Read the model definition and answer for the solid it produces. Units are mm, in the model's axes. Face numbers are marked on the shaded views. A direction names the side the tool comes from. Coordinates: 2 decimals unless noted, no trailing zeros. Write each loop counter-clockwise with the first axis right and the second up, starting at its lowest first coordinate (ties: lowest second). Pieces come first, ordered by that corner, then holes.
1) Determine the mould class of the marked faces 3, 4, 5 and 6 for opening direction X: +X half, -X half, draft (parallel to the pull), parting line (faces both ways), or undercut.
2) Find the intervals of material crossed by line 1 (X direction, y = 1.85, z = -8); line 2 (Z direction, x = 8, y = 1.75); line 3 (Z direction, x = 8, y = -2.25), in increasing order.
3) The part is cut by section D-D (z = -2.75). Determine the outline of the cut face in (x, y), then the cut area to 3 significant figures.
4) Which of the six approach directions +Z, -Z, +X, -X, +Y, -Y give full straight-line access (tool end or side, diameter ignored) to the marked faces 1 and 2?
5) The part is cut by section A-A (z = -8). Determine the outline of the cut face in (x, y), then the cut area to 3 significant figures.
6) The part is cut by section B-B (x = 8). Determine the outline of the cut face in (y, z), then the cut area to 3 significant figures.
7) This flat-tipped pin is pushed along its axis until it touches: pin 1 Ø2 at (x, z) = (5.5, -8.5) entering from +Y. Where does it stop, or does it pass through?
8) The part is cut by section C-C (y = -3.75). Determine the outline of the cut face in (x, z).
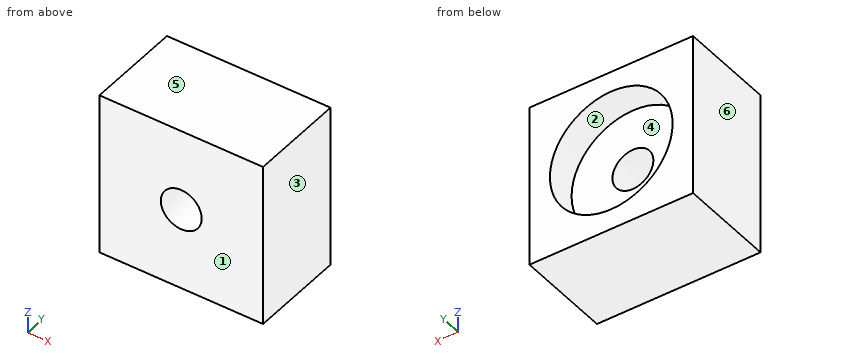
from build123d import *

# Parameters (mm, degrees)
SKETCH1_W           = 16
SKETCH1_H           = 16
SKETCH1_R           = 6
BOSS_EXTRUDE1_DEPTH = 3
SKETCH2_W           = 16
SKETCH2_H           = 16
BOSS_EXTRUDE2_DEPTH = 6.35
SKETCH3_R           = 2
CUT_EXTRUDE1_DEPTH  = 6.35


with BuildPart() as part:
    # Sketch1 → Boss-Extrude1 (new body)
    with BuildSketch(Plane(origin=(0, 0, 0), x_dir=(1, 0, 0), z_dir=(0, 1, 0))):
        with Locations((8, 8)):
            Rectangle(SKETCH1_W, SKETCH1_H)
        with Locations((8, 8)):
            Circle(SKETCH1_R, mode=Mode.SUBTRACT)
    extrude(amount=BOSS_EXTRUDE1_DEPTH)

    # Sketch2 → Boss-Extrude2 (add)
    with BuildSketch(Plane.XZ):
        with Locations((8, -8)):
            Rectangle(SKETCH2_W, SKETCH2_H)
    extrude(amount=BOSS_EXTRUDE2_DEPTH)

    # Sketch3 → Cut-Extrude1 (cut)
    with BuildSketch(Plane.XZ.offset(6.35)):
        with Locations((8, -8)):
            Circle(SKETCH3_R)
    extrude(amount=-CUT_EXTRUDE1_DEPTH, mode=Mode.SUBTRACT)


solid = part.part
Reported:
1. face 3: +X half
1. face 4: undercut
1. face 5: draft
1. face 6: -X half
2. line 1: x = 0 to 2, 14 to 16
2. line 2: z = -16 to -14, -2 to 0
2. line 3: z = -16 to -10, -6 to 0
3. outline: (0, -6.35) - (16, -6.35) - (16, 3) - (10.9, 3) - (10.9, 0) - (5.1, 0) - (5.1, 3) - (0, 3) - close
3. area: 132 mm2
4. face 1: +Z, -Z, +X, -X, -Y
4. face 2: +Y
5. outline: (0, -6.35) - (6, -6.35) - (6, 0) - (2, 0) - (2, 3) - (0, 3) - close; (10, -6.35) - (16, -6.35) - (16, 3) - (14, 3) - (14, 0) - (10, 0) - close
5. area: 88.2 mm2
6. outline: (-6.35, -16) - (3, -16) - (3, -14) - (0, -14) - (0, -10) - (-6.35, -10) - close; (-6.35, -6) - (0, -6) - (0, -2) - (3, -2) - (3, 0) - (-6.35, 0) - close
6. area: 88.2 mm2
7. pin 1: stops at y = 0
8. outline: (0, -16) - (16, -16) - (16, 0) - (0, 0) - close; hole circle Ø4 at (8, -8)
